```python
from build123d import *

# Parameters (mm, degrees)
PAD_DEPTH    = 60
SKETCH001_R  = 3
HOLE_DEPTH   = 25
SKETCH002_W  = 46
SKETCH002_H  = 60
SKETCH002_R  = 2.55
PAD001_DEPTH = 4


with BuildPart() as part:
    # Sketch → Pad (new body)
    with BuildSketch(Plane.XY):
        Polygon((-8, 0), (8, 0), (8, 128), (4.05, 128), (4.05, 115), (-4.05, 115), (-4.05, 128), (-8, 128), align=None)
    extrude(amount=PAD_DEPTH)

    # Sketch001 (on Face8 of Pad) → Hole (cut)
    with BuildSketch(Plane(origin=(-8, 0, 0), x_dir=(0, -1, 0), z_dir=(-1, 0, 0))):
        with Locations((-121.5, 30)):
            Circle(SKETCH001_R)
        with Locations((-121.5, 10)):
            Circle(SKETCH001_R)
        with Locations((-121.5, 50)):
            Circle(SKETCH001_R)
    extrude(amount=-HOLE_DEPTH, mode=Mode.SUBTRACT)

    # Sketch002 (on Face1 of Hole) → Pad001 (join)
    with BuildSketch(Plane.XZ):
        with Locations((0, 30)):
            Rectangle(SKETCH002_W, SKETCH002_H)
        with Locations((-14.5, 30)):
            Circle(SKETCH002_R, mode=Mode.SUBTRACT)
        with Locations((-14.5, 10)):
            Circle(SKETCH002_R, mode=Mode.SUBTRACT)
        with Locations((14.5, 30)):
            Circle(SKETCH002_R, mode=Mode.SUBTRACT)
        with Locations((14.5, 10)):
            Circle(SKETCH002_R, mode=Mode.SUBTRACT)
        with Locations((-14.5, 50)):
            Circle(SKETCH002_R, mode=Mode.SUBTRACT)
        with Locations((14.5, 50)):
            Circle(SKETCH002_R, mode=Mode.SUBTRACT)
    extrude(amount=-PAD001_DEPTH)


solid = part.part
```
For this review, take the finished solid that the model builds, in its own axes (mm). A direction names the side the tool comes from. Give positions to 0.01 mm unless a question says otherwise; leave off trailing zeros. Order: outer loops, then holes, each group sorted by start corner. A loop starts at its lowest first (then second) coordinate and runs counter-clockwise, first axis right, second up.
1) Take a section at A-A (z = 30). Give the boundary of the cut face in (x, y), then the cut area to 3 significant figures.
2) Take a section at D-D (y = 68.5). Give the boundary of the cut face in (x, z).
3) Insertion check: pin 1 (18 mm diameter, centred on y = 59.5, z = 19, fed in from -X); pin 2 (4.5 mm diameter, centred on x = -14, z = 41.5, fed in from +Y); pin 3 (1.5 mm diameter, centred on y = 57.5, z = 10, fed in from +X). Each pin has a flat end and moves straight along its axis. Give the tip position at first contact, or say it passes through.
4) For faces 4 (the face through (-8, 67, 30)), 5 (the face through (-6, 128, 30)), 6 (the face through (0, 115, 30)), list the 3-axis set-ups (+Z, -Z, +X, -X, +Y, -Y) from which the entire face can be reached by the end or side of a thin tool; tool diameter is ignored.
5) Wall thickness on line 1 (Z direction, x = -14.5, y = 1.5); line 2 (Z direction, x = -5.6, y = 121.5); line 3 (Y direction, x = -2.5, z = 16.5): over which ranges is each line inside the solid? List them lowest first.
6) Take a section at C-C (z = 40). Give the boundary of the cut face in (x, y).
7) The part is to be moulded in two halves that separate along X. For faces 1 (the face through (12.6, 2, 31.7)), 2 (the face through (8, 65, 30)), 3 (the face through (19, 4, 30)), say which applies: released by +X, released by -X, zero draft, split by the parting line, or undercut.
8) Take a section at B-B (x = -14.5). Give the boundary of the cut face in (y, z).
Derived:
1. outline: (-23, 0) - (-17.05, 0) - (-17.05, 4) - (-23, 4) - close; (-11.95, 0) - (11.95, 0) - (11.95, 4) - (8, 4) - (8, 118.5) - (4.05, 118.5) - (4.05, 115) - (-4.05, 115) - (-4.05, 118.5) - (-8, 118.5) - (-8, 4) - (-11.95, 4) - close; (-8, 124.5) - (-4.05, 124.5) - (-4.05, 128) - (-8, 128) - close; (4.05, 124.5) - (8, 124.5) - (8, 128) - (4.05, 128) - close; (17.05, 0) - (23, 0) - (23, 4) - (17.05, 4) - close
1. area: 1,970 mm2
2. outline: (-8, 0) - (8, 0) - (8, 60) - (-8, 60) - close
3. pin 1: stops at x = -8
3. pin 2: stops at y = 4
3. pin 3: stops at x = 8
4. face 4: +Z, -Z, -X, +Y
4. face 5: +Z, -Z, +X, -X, +Y
4. face 6: +Z, -Z, +Y
5. line 1: z = 0 to 7.45, 12.55 to 27.45, 32.55 to 47.45, 52.55 to 60
5. line 2: z = 0 to 7, 13 to 27, 33 to 47, 53 to 60
5. line 3: y = 0 to 115
6. outline: (-23, 0) - (23, 0) - (23, 4) - (8, 4) - (8, 128) - (4.05, 128) - (4.05, 115) - (-4.05, 115) - (-4.05, 128) - (-8, 128) - (-8, 4) - (-23, 4) - close
7. face 1: undercut
7. face 2: released by +X
7. face 3: zero draft
8. outline: (0, 0) - (4, 0) - (4, 7.45) - (0, 7.45) - close; (0, 12.55) - (4, 12.55) - (4, 27.45) - (0, 27.45) - close; (0, 32.55) - (4, 32.55) - (4, 47.45) - (0, 47.45) - close; (0, 52.55) - (4, 52.55) - (4, 60) - (0, 60) - close
